from build123d import *

# Parameters (mm, degrees)
SKETCH1_W                                  = 115
SKETCH1_H                                  = 115
BOSS_EXTRUDE1_DEPTH                        = 30
FILLET1_R                                  = 10
SKETCH4_W                                  = 101
SKETCH4_H                                  = 101
CUT_EXTRUDE3_DEPTH                         = 20
SKETCH7_W                                  = 90
SKETCH7_H                                  = 90
CUT_EXTRUDE5_DEPTH                         = 60
FILLET3_R                                  = 10
SKETCH8_R                                  = 3.15
CUT_EXTRUDE6_DEPTH                         = 35
MIRROR2_AT_THE_SECOND_PLANE_COPY_1_SKETC_R = 3.15
MIRROR2_AT_THE_SECOND_PLANE_COPY_1_DEPTH   = 35
SKETCH11_W                                 = 40
SKETCH11_H                                 = 90
CUT_EXTRUDE9_DEPTH                         = 11
SKETCH13_W                                 = 2.5
SKETCH13_H                                 = 90
BOSS_EXTRUDE2_DEPTH                        = 17
FILLET6_R                                  = 2
SKETCH14_W                                 = 20
SKETCH14_H                                 = 30
CUT_EXTRUDE10_DEPTH                        = 11
SKETCH15_W                                 = 10
SKETCH15_H                                 = 2.5
BOSS_EXTRUDE3_DEPTH                        = 19
FILLET7_R                                  = 2
SKETCH16_W                                 = 115
SKETCH16_H                                 = 115
CUT_EXTRUDE12_DEPTH                        = 25
SKETCH17_W                                 = 10
SKETCH17_H                                 = 80
CUT_EXTRUDE13_DEPTH                        = 15
SKETCH20_R                                 = 2.25
CUT_EXTRUDE14_DEPTH                        = 25
MIRROR8_AT_THE_SECOND_PLANE_COPY_1_SKETC_R = 2.25
MIRROR8_AT_THE_SECOND_PLANE_COPY_1_DEPTH   = 25
SKETCH21_R                                 = 1.75
CUT_EXTRUDE15_DEPTH                        = 20
MIRROR9_AT_THE_SECOND_PLANE_COPY_1_SKETC_R = 1.75
MIRROR9_AT_THE_SECOND_PLANE_COPY_1_DEPTH   = 20
SKETCH24_W                                 = 15
SKETCH24_H                                 = 25
CUT_EXTRUDE16_DEPTH                        = 7
MIRROR10_AT_THE_SECOND_PLANE_COPY_1_SKET_W = 15
MIRROR10_AT_THE_SECOND_PLANE_COPY_1_SKET_H = 25
MIRROR10_AT_THE_SECOND_PLANE_COPY_1_DEPTH  = 7
SKETCH25_R                                 = 4
CUT_EXTRUDE17_DEPTH                        = 7.5
MIRROR11_AT_THE_SECOND_PLANE_COPY_1_SKET_R = 4
MIRROR11_AT_THE_SECOND_PLANE_COPY_1_DEPTH  = 7.5
SKETCH28_W                                 = 15
SKETCH28_H                                 = 14
CUT_EXTRUDE20_DEPTH                        = 20
MIRROR12_AT_THE_SECOND_PLANE_COPY_1_SKET_W = 15
MIRROR12_AT_THE_SECOND_PLANE_COPY_1_SKET_H = 14
MIRROR12_AT_THE_SECOND_PLANE_COPY_1_DEPTH  = 20
FILLET8_R                                  = 2


with BuildPart() as part:
    # Sketch1 → Boss-Extrude1 (new, symmetric)
    with BuildSketch(Plane.XY):
        Rectangle(SKETCH1_W, SKETCH1_H)
    extrude(amount=BOSS_EXTRUDE1_DEPTH, both=True)

    # Fillet1
    fillet1_edges = [part.edges().sort_by_distance(p)[0] for p in [
        (-57.5, 57.5, 0),
        (57.5, 57.5, 0),
        (57.5, -57.5, 0),
        (-57.5, -57.5, 0),
    ]]
    fillet(fillet1_edges, radius=FILLET1_R)

    # Sketch4 → Cut-Extrude3 (cut)
    with BuildSketch(Plane.XY.offset(30)):
        Rectangle(SKETCH4_W, SKETCH4_H)
    extrude(amount=-CUT_EXTRUDE3_DEPTH, mode=Mode.SUBTRACT)

    # Sketch7 → Cut-Extrude5 (cut)
    with BuildSketch(Plane.XY.offset(10)):
        Rectangle(SKETCH7_W, SKETCH7_H)
    extrude(amount=-CUT_EXTRUDE5_DEPTH, mode=Mode.SUBTRACT)

    # Fillet3
    fillet3_edges = [part.edges().sort_by_distance(p)[0] for p in [
        (-45, -45, -10),
        (-45, 45, -10),
        (45, 45, -10),
        (45, -45, -10),
    ]]
    fillet(fillet3_edges, radius=FILLET3_R)

    # Sketch8 → Cut-Extrude6 (cut)
    with BuildSketch(Plane(origin=(0, 0, -30), x_dir=(-1, 0, 0), z_dir=(0, 0, -1))):
        with Locations((-48, 48)):
            Circle(SKETCH8_R)
    cut_extrude6 = extrude(amount=-CUT_EXTRUDE6_DEPTH, mode=Mode.SUBTRACT)

    # Mirror2: Cut-Extrude6 across plane
    add(cut_extrude6.mirror(Plane.ZX), mode=Mode.SUBTRACT)

    # Mirror2 at the second plane: Cut-Extrude6 across plane
    add(cut_extrude6.mirror(Plane(origin=(0, 0, 0), x_dir=(0, 0, 1), z_dir=(1, 0, 0))), mode=Mode.SUBTRACT)

    # Mirror2 at the second plane copy 1 sketc → Mirror2 at the second plane copy 1 (cut)
    with BuildSketch(Plane(origin=(0, 0, -30), x_dir=(1, 0, 0), z_dir=(0, 0, -1))):
        with Locations((-48, 48)):
            Circle(MIRROR2_AT_THE_SECOND_PLANE_COPY_1_SKETC_R)
    extrude(amount=-MIRROR2_AT_THE_SECOND_PLANE_COPY_1_DEPTH, mode=Mode.SUBTRACT)

    # Sketch11 → Cut-Extrude9 (cut)
    with BuildSketch(Plane(origin=(57.5, 0, 0), x_dir=(0, 0, -1), z_dir=(1, 0, 0))):
        with Locations((-30, 0)):
            Rectangle(SKETCH11_W, SKETCH11_H)
    extrude(amount=-CUT_EXTRUDE9_DEPTH, mode=Mode.SUBTRACT)

    # Sketch13 → Boss-Extrude2 (add)
    with BuildSketch(Plane(origin=(57.5, 0, 0), x_dir=(0, 0, -1), z_dir=(1, 0, 0))):
        with Locations((-8.75, 0)):
            Rectangle(SKETCH13_W, SKETCH13_H)
        Polygon((-7.5, -45), (-10, -45), (-30, -45), (-30, -47.5), (-7.5, -47.5), align=None)
        Polygon((-30, 45), (-10, 45), (-7.5, 45), (-7.5, 47.5), (-30, 47.5), align=None)
    extrude(amount=BOSS_EXTRUDE2_DEPTH)

    # Fillet6
    fillet6_edges = [part.edges().sort_by_distance(p)[0] for p in [
        (62.5, 45, 10),
        (62.5, -45, 10),
        (66, -47.5, 7.5),
        (66, 47.5, 7.5),
    ]]
    fillet(fillet6_edges, radius=FILLET6_R)

    # Sketch14 → Cut-Extrude10 (cut)
    with BuildSketch(Plane.ZY.offset(57.5)):
        with Locations((30, 0)):
            Rectangle(SKETCH14_W, SKETCH14_H)
    extrude(amount=-CUT_EXTRUDE10_DEPTH, mode=Mode.SUBTRACT)

    # Sketch15 → Boss-Extrude3 (add)
    with BuildSketch(Plane.ZY.offset(57.5)):
        Polygon((20, -15), (20, 15), (20, 17.5), (17.5, 17.5), (17.5, -17.5), (20, -17.5), align=None)
        with Locations((25, 16.25)):
            Rectangle(SKETCH15_W, SKETCH15_H)
        with Locations((25, -16.25)):
            Rectangle(SKETCH15_W, SKETCH15_H)
    extrude(amount=BOSS_EXTRUDE3_DEPTH)

    # Fillet7
    fillet7_edges = [part.edges().sort_by_distance(p)[0] for p in [
        (-63.5, -15, 20),
        (-63.5, 15, 20),
        (-67, 17.5, 17.5),
        (-67, -17.5, 17.5),
    ]]
    fillet(fillet7_edges, radius=FILLET7_R)

    # Sketch16 → Cut-Extrude12 (cut)
    with BuildSketch(Plane(origin=(0, 0, -30), x_dir=(-1, 0, 0), z_dir=(0, 0, -1))):
        Rectangle(SKETCH16_W, SKETCH16_H)
    extrude(amount=-CUT_EXTRUDE12_DEPTH, mode=Mode.SUBTRACT)

    # Sketch17 → Cut-Extrude13 (cut)
    with BuildSketch(Plane(origin=(0, 0, 7.5), x_dir=(-1, 0, 0), z_dir=(0, 0, -1))):
        with Locations((-62.5, 0)):
            Rectangle(SKETCH17_W, SKETCH17_H)
    extrude(amount=-CUT_EXTRUDE13_DEPTH, mode=Mode.SUBTRACT)

    # Sketch20 → Cut-Extrude14 (cut)
    with BuildSketch(Plane(origin=(57.5, 0, 0), x_dir=(0, 0, -1), z_dir=(1, 0, 0))):
        with Locations((0, 30)):
            Circle(SKETCH20_R)
    cut_extrude14 = extrude(amount=-CUT_EXTRUDE14_DEPTH, mode=Mode.SUBTRACT)

    # Mirror8: Cut-Extrude14 across plane
    add(cut_extrude14.mirror(Plane(origin=(0, 0, 0), x_dir=(0, 0, 1), z_dir=(1, 0, 0))), mode=Mode.SUBTRACT)

    # Mirror8 at the second plane: Cut-Extrude14 across plane
    add(cut_extrude14.mirror(Plane.ZX), mode=Mode.SUBTRACT)

    # Mirror8 at the second plane copy 1 sketc → Mirror8 at the second plane copy 1 (cut)
    with BuildSketch(Plane(origin=(-57.5, 0, 0), x_dir=(0, 0, -1), z_dir=(-1, 0, 0))):
        with Locations((0, 30)):
            Circle(MIRROR8_AT_THE_SECOND_PLANE_COPY_1_SKETC_R)
    extrude(amount=-MIRROR8_AT_THE_SECOND_PLANE_COPY_1_DEPTH, mode=Mode.SUBTRACT)

    # Sketch21 → Cut-Extrude15 (cut)
    with BuildSketch(Plane.XY.offset(30)):
        with Locations((30, 54)):
            Circle(SKETCH21_R)
    cut_extrude15 = extrude(amount=-CUT_EXTRUDE15_DEPTH, mode=Mode.SUBTRACT)

    # Mirror9: Cut-Extrude15 across plane
    add(cut_extrude15.mirror(Plane.ZX), mode=Mode.SUBTRACT)

    # Mirror9 at the second plane: Cut-Extrude15 across plane
    add(cut_extrude15.mirror(Plane(origin=(0, 0, 0), x_dir=(0, 0, 1), z_dir=(1, 0, 0))), mode=Mode.SUBTRACT)

    # Mirror9 at the second plane copy 1 sketc → Mirror9 at the second plane copy 1 (cut)
    with BuildSketch(Plane(origin=(0, 0, 30), x_dir=(-1, 0, 0), z_dir=(0, 0, 1))):
        with Locations((30, 54)):
            Circle(MIRROR9_AT_THE_SECOND_PLANE_COPY_1_SKETC_R)
    extrude(amount=-MIRROR9_AT_THE_SECOND_PLANE_COPY_1_DEPTH, mode=Mode.SUBTRACT)

    # Sketch24 → Cut-Extrude16 (cut)
    with BuildSketch(Plane(origin=(0, 57.5, 0), x_dir=(1, 0, 0), z_dir=(0, 1, 0))):
        with Locations((30, -12.5)):
            Rectangle(SKETCH24_W, SKETCH24_H)
    cut_extrude16 = extrude(amount=-CUT_EXTRUDE16_DEPTH, mode=Mode.SUBTRACT)

    # Mirror10: Cut-Extrude16 across plane
    add(cut_extrude16.mirror(Plane(origin=(0, 0, 0), x_dir=(0, 0, 1), z_dir=(1, 0, 0))), mode=Mode.SUBTRACT)

    # Mirror10 at the second plane: Cut-Extrude16 across plane
    add(cut_extrude16.mirror(Plane.ZX), mode=Mode.SUBTRACT)

    # Mirror10 at the second plane copy 1 sket → Mirror10 at the second plane copy 1 (cut)
    with BuildSketch(Plane(origin=(0, -57.5, 0), x_dir=(-1, 0, 0), z_dir=(0, -1, 0))):
        with Locations((30, -12.5)):
            Rectangle(MIRROR10_AT_THE_SECOND_PLANE_COPY_1_SKET_W, MIRROR10_AT_THE_SECOND_PLANE_COPY_1_SKET_H)
    extrude(amount=-MIRROR10_AT_THE_SECOND_PLANE_COPY_1_DEPTH, mode=Mode.SUBTRACT)

    # Sketch25 → Cut-Extrude17 (cut)
    with BuildSketch(Plane.ZY.offset(-45)):
        with Locations((0, 30)):
            Circle(SKETCH25_R)
    cut_extrude17 = extrude(amount=-CUT_EXTRUDE17_DEPTH, mode=Mode.SUBTRACT)

    # Mirror11: Cut-Extrude17 across plane
    add(cut_extrude17.mirror(Plane.ZX), mode=Mode.SUBTRACT)

    # Mirror11 at the second plane: Cut-Extrude17 across plane
    add(cut_extrude17.mirror(Plane(origin=(0, 0, 0), x_dir=(0, 0, 1), z_dir=(1, 0, 0))), mode=Mode.SUBTRACT)

    # Mirror11 at the second plane copy 1 sket → Mirror11 at the second plane copy 1 (cut)
    with BuildSketch(Plane(origin=(-45, 0, 0), x_dir=(0, 0, 1), z_dir=(1, 0, 0))):
        with Locations((0, 30)):
            Circle(MIRROR11_AT_THE_SECOND_PLANE_COPY_1_SKET_R)
    extrude(amount=-MIRROR11_AT_THE_SECOND_PLANE_COPY_1_DEPTH, mode=Mode.SUBTRACT)

    # Sketch28 → Cut-Extrude20 (cut)
    with BuildSketch(Plane(origin=(0, 0, -5), x_dir=(-1, 0, 0), z_dir=(0, 0, -1))):
        with Locations((-30, 57.5)):
            Rectangle(SKETCH28_W, SKETCH28_H)
    cut_extrude20 = extrude(amount=-CUT_EXTRUDE20_DEPTH, mode=Mode.SUBTRACT)

    # Mirror12: Cut-Extrude20 across plane
    add(cut_extrude20.mirror(Plane.ZX), mode=Mode.SUBTRACT)

    # Mirror12 at the second plane: Cut-Extrude20 across plane
    add(cut_extrude20.mirror(Plane(origin=(0, 0, 0), x_dir=(0, 0, 1), z_dir=(1, 0, 0))), mode=Mode.SUBTRACT)

    # Mirror12 at the second plane copy 1 sket → Mirror12 at the second plane copy 1 (cut)
    with BuildSketch(Plane(origin=(0, 0, -5), x_dir=(1, 0, 0), z_dir=(0, 0, -1))):
        with Locations((-30, 57.5)):
            Rectangle(MIRROR12_AT_THE_SECOND_PLANE_COPY_1_SKET_W, MIRROR12_AT_THE_SECOND_PLANE_COPY_1_SKET_H)
    extrude(amount=-MIRROR12_AT_THE_SECOND_PLANE_COPY_1_DEPTH, mode=Mode.SUBTRACT)

    # Fillet8
    fillet8_edges = [part.edges().sort_by_distance(p)[0] for p in [
        (37.5, 50.5, 2.5),
        (22.5, 50.5, 2.5),
        (37.5, 57.5, 10),
        (22.5, 57.5, 10),
        (37.5, -57.5, 10),
        (22.5, -57.5, 10),
        (22.5, -50.5, 2.5),
        (37.5, -50.5, 2.5),
        (-37.5, 57.5, 10),
        (-22.5, 57.5, 10),
        (-22.5, 50.5, 2.5),
        (-37.5, 50.5, 2.5),
        (-37.5, -50.5, 2.5),
        (-22.5, -50.5, 2.5),
        (-37.5, -57.5, 10),
        (-22.5, -57.5, 10),
    ]]
    fillet(fillet8_edges, radius=FILLET8_R)


solid = part.part
Read the model definition and answer for the solid it produces. Units are mm, in the model's axes. A direction names the side the tool comes from. Give positions to 0.01 mm unless a question says otherwise; leave off trailing zeros. Write each loop counter-clockwise with the first axis right and the second up, starting at its lowest first coordinate (ties: lowest second). Pieces come first, ordered by that corner, then holes. Notation, with made-up numbers: (64, 34) - (69, 34) arc R35 ccw to (69, 72) - close; hole circle Ø8 at (25.5, 48). An arc over 180 degrees is marked (long way). Return JSON: item names as keys, results as strings.
Q1. Given P1, Ø1.9, axis at x = 47, y = 46.5, coming from the -Z side; P2, Ø9, axis at y = 31.5, z = 0, coming from the +X side; P3, Ø5, axis at x = -49, y = 48.5, coming from the -Z side; P4, Ø1.5, axis at y = 54, z = 15, coming from the +X side, each flat-ended and moving along its own axis, determine where each tip first touches the part or whether it passes through.
Reply:
{"P1": "z = 5", "P2": "x = 57.5", "P3": "z = -5", "P4": "x = 55.68"}
Q2. For faces 4 (the face through (-67, 17.5, 25)), 5 (the face through (48.698, -33.966, -0.521)), 6 (the face through (45, 0, 3)), 7 (the face through (-50.5, -1, 18)), determine the directions among +Z, -Z, +X, -X, +Y, -Y from which every point of the face is accessible in a straight line to the end or side of a thin tool.
Reply:
{"face 4": "+Z, -Z, -X, +Y", "face 5": "none", "face 6": "+Z, -Z", "face 7": "+Z"}
Q3. A cutting plane is placed at C-C, the plane y = 23.5. Determine the outline of the cut face in (x, z).
Reply:
{"outline": "(-57.5, -5) - (-45, -5) - (-45, 10) - (-50.5, 10) - (-50.5, 30) - (-57.5, 30) - close; (45, -5) - (57.5, -5) - (57.5, 10) - (45, 10) - close; (67.5, 7.5) - (74.5, 7.5) - (74.5, 10) - (67.5, 10) - close"}
Q4. A cutting plane is placed at B-B, the plane x = 30. Determine the outline of the cut face in (y, z), and give its area (3 significant figures).
Reply:
{"outline": "(-57.5, 25) - (-55.75, 25) - (-55.75, 30) - (-57.5, 30) - close; (-52.25, 25) - (-50.5, 25) - (-50.5, 30) - (-52.25, 30) - close; (-50.5, -5) - (-45, -5) - (-45, 10) - (-50.5, 10) - close; (45, -5) - (50.5, -5) - (50.5, 10) - (45, 10) - close; (50.5, 25) - (52.25, 25) - (52.25, 30) - (50.5, 30) - close; (55.75, 25) - (57.5, 25) - (57.5, 30) - (55.75, 30) - close", "area": "200 mm²"}
Q5. A cutting plane is placed at A-A, the plane y = -30. Count the separate pieces of the cut face and the enclosed holes in it, and give its area (4 significant figures).
Reply:
{"separate pieces": "5", "enclosed holes": "0", "area": "367.5 mm²"}
Q6. For a pull along Y with two mould halves and no side action, classify faces 1 (the face through (28.61, -52.94, 27.54)), 2 (the face through (-32, 54, 25)), 3 (the face through (-1, -57.5, 13)) as released by +Y, released by -Y, zero draft, split by the parting line, or undercut.
Reply:
{"face 1": "undercut", "face 2": "zero draft", "face 3": "released by -Y"}
Q7. A cutting plane is placed at D-D, the plane x = -2. Determine the outline of the cut face in (y, z), and give its area (3 significant figures).
Reply:
{"outline": "(-57.5, -5) - (-45, -5) - (-45, 10) - (-50.5, 10) - (-50.5, 30) - (-57.5, 30) - close; (45, -5) - (57.5, -5) - (57.5, 30) - (50.5, 30) - (50.5, 10) - (45, 10) - close", "area": "655 mm²"}
Q8. Consider line 1 along X through (y, z) = (-34, 9.5); line 2 along Y through (x, z) = (23, -2); line 3 along X through (y, z) = (32.5, -1). Determine where each line is inside the solid, lowest interval first. Write a range as [from, to].
Reply:
{"line 1": "[-57.5, -45], [45, 57.5], [67.5, 74.5]", "line 2": "[-51.18, -45], [45, 51.18]", "line 3": "[-57.5, -52.5], [52.5, 57.5]"}
